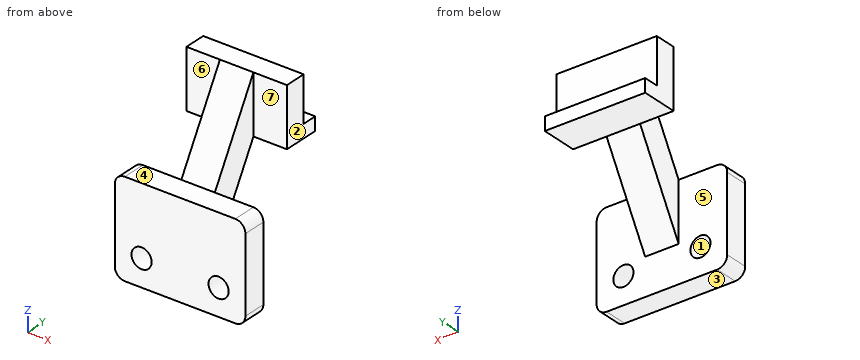
from build123d import *

# Parameters (mm, degrees)
ESTRUSIONE_ESTRUSIONE1_DEPTH = 78
TAGLIO_ESTRUSIONE1_DEPTH     = 29
TAGLIO_ESTRUSIONE2_DEPTH     = 29
SCHIZZO4_W                   = 35
SCHIZZO4_H                   = 22
TAGLIO_ESTRUSIONE3_DEPTH     = 9
SCHIZZO5_W                   = 35
SCHIZZO5_H                   = 22
TAGLIO_ESTRUSIONE4_DEPTH     = 9
SCHIZZO6_R                   = 6
TAGLIO_ESTRUSIONE5_DEPTH     = 144.738003889
RACCORDO1_R                  = 6


with BuildPart() as part:
    # Schizzo1 → Estrusione-Estrusione1 (new body)
    with BuildSketch(Plane(origin=(0, 0, 0), x_dir=(0, 0, -1), z_dir=(1, 0, 0))):
        Polygon((-57, 0), (0, 0), (0, 14), (-22, 14), (-73.961524227, 44), (-73.961524227, 66), (-81.961524227, 66), (-81.961524227, 57), (-108.961524227, 57), (-108.961524227, 44), (-57, 14), align=None)
    extrude(amount=-ESTRUSIONE_ESTRUSIONE1_DEPTH)

    # Schizzo2 → Taglio-Estrusione1 (cut)
    with BuildSketch(Plane(origin=(0, 0, 0), x_dir=(0, 0, -1), z_dir=(1, 0, 0))):
        Polygon((-22, 14), (-57, 14), (-108.961524227, 44), (-73.961524227, 44), align=None)
    extrude(amount=-TAGLIO_ESTRUSIONE1_DEPTH, mode=Mode.SUBTRACT)

    # Schizzo3 → Taglio-Estrusione2 (cut)
    with BuildSketch(Plane.ZY.offset(78)):
        Polygon((57, 14), (22, 14), (73.961524227, 44), (108.961524227, 44), align=None)
    extrude(amount=-TAGLIO_ESTRUSIONE2_DEPTH, mode=Mode.SUBTRACT)

    # Schizzo4 → Taglio-Estrusione3 (cut)
    with BuildSketch(Plane.ZY.offset(78)):
        with Locations((91.461524227, 55)):
            Rectangle(SCHIZZO4_W, SCHIZZO4_H)
    extrude(amount=-TAGLIO_ESTRUSIONE3_DEPTH, mode=Mode.SUBTRACT)

    # Schizzo5 → Taglio-Estrusione4 (cut)
    with BuildSketch(Plane(origin=(0, 0, 0), x_dir=(0, 0, -1), z_dir=(1, 0, 0))):
        with Locations((-91.461524227, 55)):
            Rectangle(SCHIZZO5_W, SCHIZZO5_H)
    extrude(amount=-TAGLIO_ESTRUSIONE4_DEPTH, mode=Mode.SUBTRACT)

    # Schizzo6 → Taglio-Estrusione5 (cut, through all)
    with BuildSketch(Plane(origin=(0, 14, 0), x_dir=(1, 0, 0), z_dir=(0, 1, 0))):
        with Locations(Location((-16, -16, 0), (0, 0, 270))):
            Circle(SCHIZZO6_R)
        with Locations(Location((-62, -16, 0), (0, 0, 270))):
            Circle(SCHIZZO6_R)
    extrude(amount=-TAGLIO_ESTRUSIONE5_DEPTH, mode=Mode.SUBTRACT)

    # Raccordo1
    raccordo1_edges = [part.edges().sort_by_distance(p)[0] for p in [
        (0, 7, 0),
        (0, 7, 57),
        (-78, 7, 57),
        (-78, 7, 0),
    ]]
    fillet(raccordo1_edges, radius=RACCORDO1_R)


solid = part.part
Verification items for the finished model (mm, model axes). Face numbers are marked on the shaded views. A direction names the side the tool comes from. Round coordinates to 2 decimals unless told otherwise and drop trailing zeros. Order: outer loops, then holes, each group sorted by start corner. A loop starts at its lowest first (then second) coordinate and runs counter-clockwise, first axis right, second up.
1. Access from +Z, -Z, +X, -X, +Y, -Y to the whole of each face (thin tool, end or side, straight path). Record for the marked faces 4, 5, 6 and 7.
Final values:
face 4: +Z, +X, -X, -Y
face 5: -Z, +Y
face 6: +Z, -Z, -X, -Y
face 7: +Z, -Z, +X, -Y
2. Section check C-C on x = -24. Record the cut outline in (y, z).
Final values:
outline: (0, 0) - (14, 0) - (14, 57) - (0, 57) - close; (44, 73.96) - (66, 73.96) - (66, 81.96) - (57, 81.96) - (57, 108.96) - (44, 108.96) - close
3. Section check A-A on x = -16. Record the cut outline in (y, z), then the cut area to 3 significant figures.
Final values:
outline: (0, 0) - (14, 0) - (14, 10) - (0, 10) - close; (0, 22) - (14, 22) - (14, 57) - (0, 57) - close; (44, 73.96) - (66, 73.96) - (66, 81.96) - (57, 81.96) - (57, 108.96) - (44, 108.96) - close
area: 1,160 mm2
4. Section check D-D on y = 9.5. Record the cut outline in (x, z).
Final values:
outline: (-78, 6) arc R6 ccw to (-72, 0) - (-6, 0) arc R6 ccw to (0, 6) - (0, 51) arc R6 ccw to (-6, 57) - (-72, 57) arc R6 ccw to (-78, 51) - close; hole circle Ø12 at (-62, 16); hole circle Ø12 at (-16, 16)
5. Release check for a two-part mould opening along X. For the marked faces 1, 2 and 3 record: +X half, -X half, draft (parallel to the pull), parting line (faces both ways), or undercut.
Final values:
face 1: undercut
face 2: +X half
face 3: draft
6. Go/stop test with flat-tipped pins: P1, Ø4.5, axis at x = -48, y = 61.5, coming from the +Z side; P2, Ø17.5, axis at y = 52, z = 85.5, coming from the -X side; P3, Ø21.5, axis at x = -40, z = 101.5, coming from the +Y side; P4, Ø24, axis at y = 22.5, z = 57, coming from the -X side. Record where each tip stops, or that it passes through.
Final values:
P1: stops at z = 81.96
P2: stops at x = -69
P3: stops at y = 57
P4: stops at x = -78
7. Section check B-B on z = 16. Record the cut outline in (x, y), then the cut area to 3 significant figures.
Final values:
outline: (-78, 0) - (-68, 0) - (-68, 14) - (-78, 14) - close; (-56, 0) - (-22, 0) - (-22, 14) - (-56, 14) - close; (-10, 0) - (0, 0) - (0, 14) - (-10, 14) - close
area: 756 mm2
8. Thickness scan on L1, parallel to X at y = 9, z = 16; L2, parallel to Y at x = -65, z = 100; L3, parallel to Y at x = -51, z = 51. Record the ranges inside material, lowest first.
Final values:
L1: x = -78 to -68, -56 to -22, -10 to 0
L2: y = 44 to 57
L3: y = 0 to 14
